Autodesk Inventor part; units mm, degrees
ref_plane "Work Plane2" through (2.032, 0, 0) normal (0, 1, 0) x (1, 0, 0)
ref_plane "YZ Plane" through (0, 0, 0) normal (1, 0, 0) x (0, 1, 0)
ref_plane "XZ Plane" through (0, 0, 0) normal (0, 1, 0) x (-1, 0, 0)
sketch "Эскиз1" plane through (0, 0, 0) normal (0, 0, 1) x (1, 0, 0)
  line L0 (2.28, 0) -> (10, 0)
  line L1 (10, 0) -> (10, 1.5)
  line L2 (10, 1.5) -> (1.7, 1.5)
  line L3 (0.6, 2.6) -> (0, 2.6)
  line L4 (-2, 0) -> (12, 0)
  line L5 (0, -0.52) -> (0, 3.12)
  line L6 (0, 1.625) -> (1.9268, 0.6644)
  line L7 (1.9268, 0.6644) -> (2.28, 0)
  line L8 (1.7, 1.5) -> (0.6, 2.6)
  line L9 (0, 2.6) -> (0, 1.625)
  dimension "d2" = 3
  dimension "d3" = 5.2
  dimension "d4" = 2.28
  dimension "d5" = 3.25
  dimension "d6" = 26.5
  dimension "d7" = 62
  dimension "d13" = 45
  dimension "d14" = 1.7
  dimension "d15" = 10
revolve "Базовый элемент" add sketch "Эскиз1" angle 360 about axis through (2.28, 0, 0) along (1, 0, 0) contours L7 L6 L5 L3 L8 L2 L1 L0
sketch "Эскиз2" plane through (0, 0, 0) normal (-1, 0, 0) x (0, 0, 1)
  line L0 (0, -3.64) -> (0, 3.64)
  line L1 (-3.64, 0) -> (3.64, 0)
  line L2 (0, 1.625) -> (0, 0) construction
  line L3 (0, 0) -> (1.625, 0) construction
  arc A0 (0.5417, 0) -> (0, 0.5417) centre (0, 0) ccw
  line L4 (0, 0) -> (0.7947, 0.7947) construction
  arc A1 (0.8125, 0) -> (0, 0.8125) centre (0, 0) ccw construction
  line L5 (0.395, 1.5763) -> (0.2593, 0.77)
  line L6 (1.5763, 0.395) -> (0.77, 0.2593)
  arc A2 (0.2593, 0.77) -> (0.77, 0.2593) centre (0.6964, 0.6964) ccw
  arc A3 (1.625, 0) -> (1.5763, 0.395) centre (0, 0) ccw
  arc A4 (0.395, 1.5763) -> (0, 1.625) centre (0, 0) ccw
  arc A5 (1.5763, 0.395) -> (0.395, 1.5763) centre (0, 0) ccw
  line L7 (0.395, -1.5763) -> (0.2593, -0.77)
  line L8 (1.5763, -0.395) -> (0.77, -0.2593)
  arc A6 (0.77, -0.2593) -> (0.2593, -0.77) centre (0.6964, -0.6964) ccw
  arc A7 (1.5763, -0.395) -> (1.625, 0) centre (0, 0) ccw
  arc A8 (0, -1.625) -> (0.395, -1.5763) centre (0, 0) ccw
  arc A9 (0.395, -1.5763) -> (1.5763, -0.395) centre (0, 0) ccw
  line L9 (-0.395, 1.5763) -> (-0.2593, 0.77)
  line L10 (-1.5763, 0.395) -> (-0.77, 0.2593)
  arc A10 (-0.77, 0.2593) -> (-0.2593, 0.77) centre (-0.6964, 0.6964) ccw
  arc A11 (-1.5763, 0.395) -> (-1.625, 0) centre (0, 0) ccw
  arc A12 (0, 1.625) -> (-0.395, 1.5763) centre (0, 0) ccw
  arc A13 (-0.395, 1.5763) -> (-1.5763, 0.395) centre (0, 0) ccw
  arc A14 (-1.5763, -0.395) -> (-0.395, -1.5763) centre (0, 0) ccw
  arc A15 (-0.395, -1.5763) -> (0, -1.625) centre (0, 0) ccw
  arc A16 (-1.625, 0) -> (-1.5763, -0.395) centre (0, 0) ccw
  line L11 (-1.5763, -0.395) -> (-0.77, -0.2593)
  arc A17 (-0.2593, -0.77) -> (-0.77, -0.2593) centre (-0.6964, -0.6964) ccw
  line L12 (-0.395, -1.5763) -> (-0.2593, -0.77)
  dimension "d18" = 45
  dimension "d19" = 1.0833
  dimension "d20" = 1.625
  dimension "d21" = 3.25
  dimension "d22" = 0.395
extrude "Паз" add sketch "Эскиз2" against normal up to next contours A2 L5 A5 L6 | L9 A10 L10 A13 | L7 A6 L8 A9 | A14 L11 A17 L12
fillet "Сопряжение1" radius 0.158 4 edges at (0, 1.625, 0) (0, 0, 1.625) (0, -1.625, 0) (0, 0, -1.625)
thread "Резьба"
chamfer "Фаска1" distance 0.44 distance2 0.3067 1 edges at (10, -1.5, 0) measured on face at (10, 0.3743, 0.3316)
ref_plane "Work Plane2" through (2.032, 0, 0) normal (0, 1, 0) x (1, 0, 0)
equation "\"d2\" = GD"
equation "\"d3\" = KOD"
equation "\"d4\" = INTI"
equation "\"d5\" = SDM"
equation "\"d13\" = 0.5 * SEWI"
equation "\"d14\" = KOH"
equation "\"d15\" = NLG"
equation "\"d19\" = 0.333333 * SDM"
equation "\"d20\" = 0.5 * SDM"
equation "\"d21\" = SDM"
equation "\"d22\" = 0.5 * SBR"
equation "\"d45\" = INTI"
equation "\"d25\" = 0.2 * SBR"
equation "\"d9\" = GEL"
equation "\"d11\" = -0.5 * SPD + 0.5 * GD"
equation "\"d12\" = GUL"
equation "\"GD\" = NND"
equation "\"NLG\" = 10"
equation "\"GEL\" = 7.1"
equation "\"KOD\" = 5.2"
equation "\"KOH\" = 1.7"
equation "\"SDM\" = 3.25"
equation "\"INTI\" = 2.28"
equation "\"SBR\" = 0.79"
equation "\"GUL\" = 0.61345 * PTC"
equation "\"SPD\" = 2.12"
equation "\"SEWI\" = 90deg"
equation "\"d1\" = KOH"
equation "\"d17\" = SDM"
equation "\"TOA\" = 30deg"
equation "\"KODMAX\" = 6.3"
equation "\"EPV\" = 3.15"
equation "\"THREADDIA\" = 3"
equation "\"BDM\" = 3"
equation "\"PTC\" = 0.5"
equation "\"NND\" = 3"
equation "\"GAL\" = 0.61345 * PTC"
equation "\"GD1\" = THREADDIA - 1.2269 * PTC"
properties part number "IFI 513 - M3x0,5 x 10, CRFCHMSTIM(1)" material "Сталь, мягкая"
Design review of the part built by this model. Coordinates are the model's own, in mm. A direction names the side the tool comes from. Give positions to 0.01 mm unless a question says otherwise; leave off trailing zeros. Order: outer loops, then holes, each group sorted by start corner. A loop starts at its lowest first (then second) coordinate and runs counter-clockwise, first axis right, second up. Notation, with made-up numbers: (-21.75, 0) - (-17.75, 0) arc R33 cw to (-17.75, 39) - close; hole circle Ø10 at (2.25, 54). An arc over 180 degrees is marked (long way). Use CSV: the item, a comma, the result in double quotes. Start each with the question number.
Q1. Draft analysis for pull direction Y (two halves, no side actions). For faces 1 (the face through (0, 1, -1)), 2 (the face through (0.99, 1.13, 0.01)), 3 (the face through (5.64, -1.5, -0.07)), state which applies: pulls with the +Y half, pulls with the -Y half, needs draft (parallel to the pull), parting line crosses it, or undercut.
Q2. Take a section at A-A (x = 3.75). State the section outline as (y, z) points, and give its area (3 significant figures).
Q3. Machinability: for faces 4 (the face through (0.4, -1, -0.3)), 5 (the face through (10, 0, 0)), which of the approach directions +Z, -Z, +X, -X, +Y, -Y give a long, thin tool a straight path to every point of the face, cutting with its end or side? Answer none if there is none.
Q4. For P1, Ø2, axis at x = 8, z = 0, coming from the -Y side, flat-tipped, find the tip position at first contact; note if it passes through.
Q5. For line 1 (Y direction, x = 0.5, z = 0.15); line 2 (X direction, y = -0.9, z = 1.4); line 3 (Y direction, x = 1, z = -1.5), list the stretches that pass through material, from the lowest coordinate up.
Calculated:
1,face 1,"needs draft"
1,face 2,"undercut"
1,face 3,"parting line crosses it"
2,outline,"circle Ø3 at (0, 0)"
2,area,"7.07 mm²"
3,face 4,"-X"
3,face 5,"+Z, -Z, +X, +Y, -Y"
4,P1,"stops at y = -1.5"
5,line 1,"y = -2.6 to -1.37, 1.37 to 2.6"
5,line 2,"x = 0 to 1.54"
5,line 3,"y = -1.61 to 1.61"
